Check sheet for the modelled part. Datum: model origin and axes. Units: mm. A direction names the side the tool comes from. Round coordinates to 2 decimals unless told otherwise and drop trailing zeros. Loops run counter-clockwise (first coordinate to the right, second up) from the corner with the lowest first, then second, coordinate; pieces in that order, holes last. Notation, with made-up numbers: (-8, 28) - (-3, 28) arc R20 cw to (-3, 39) - close; hole circle Ø10 at (-23.5, 68.25). An arc over 180 degrees is marked (long way). Return JSON: item names as keys, results as strings.
from build123d import *

# Parameters (mm, degrees)
PAD_DEPTH           = 26
SKETCH001_R         = 1.6891
POCKET_DEPTH        = 24.5
POCKET001_DEPTH     = 1.6
POCKET002_DEPTH     = 5
POCKET004_DEPTH     = 10
LINEARPATTERN_COUNT = 8
LINEARPATTERN_PITCH = 3.714286
SKETCH009_W         = 20
SKETCH009_H         = 4.8
POCKET007_DEPTH     = 0.5
SKETCH004_W         = 17.68
SKETCH004_H         = 4.4
POCKET015_DEPTH     = 5
SKETCH013_W         = 10.6
SKETCH013_H         = 6
POCKET016_DEPTH     = 5
SKETCH014_R         = 0.5
POCKET017_DEPTH     = 5
SKETCH015_R         = 1.9685
POCKET018_DEPTH     = 5
POCKET019_DEPTH     = 5
POCKET020_DEPTH     = 10
SKETCH021_R         = 7
PAD001_DEPTH        = 9
SKETCH019_R         = 4.6
POCKET021_DEPTH     = 1.2
SKETCH018_R         = 4
POCKET022_DEPTH     = 8.5


with BuildPart() as part:
    # Sketch → Pad (new body)
    with BuildSketch(Plane.XY):
        with BuildLine():
            Line((-17, 37.5), (17, 37.5))
            ThreePointArc((21, 33.5), (19.828427, 36.328427), (17, 37.5))
            Line((21, 33.5), (21, -33.5))
            ThreePointArc((17, -37.5), (19.828427, -36.328427), (21, -33.5))
            Line((17, -37.5), (-17, -37.5))
            ThreePointArc((-21, -33.5), (-19.828427, -36.328427), (-17, -37.5))
            Line((-21, -33.5), (-21, 33.5))
            ThreePointArc((-17, 37.5), (-19.828427, 36.328427), (-21, 33.5))
        make_face()
    extrude(amount=PAD_DEPTH)

    # Sketch001 (on Face10 of Pad) → Pocket (cut)
    with BuildSketch(Plane.XY.offset(26)):
        with Locations((-16.5, -33)):
            Circle(SKETCH001_R)
        with Locations((16.5, -33)):
            Circle(SKETCH001_R)
        with Locations((16.5, 33)):
            Circle(SKETCH001_R)
        with Locations((-16.5, 33)):
            Circle(SKETCH001_R)
        with BuildLine():
            Line((-12.6, 36), (12.6, 36))
            Line((12.6, 36), (12.6, 33.1))
            ThreePointArc((12.6, 33.1), (13.771573, 30.271573), (16.6, 29.1))
            Line((16.6, 29.1), (19.5, 29.1))
            Line((19.5, 29.1), (19.5, -29.1))
            Line((19.5, -29.1), (16.6, -29.1))
            ThreePointArc((16.6, -29.1), (13.771573, -30.271573), (12.6, -33.1))
            Line((12.6, -33.1), (12.6, -36))
            Line((12.6, -36), (-12.6, -36))
            Line((-12.6, -36), (-12.6, -33.1))
            ThreePointArc((-12.6, -33.1), (-13.771573, -30.271573), (-16.6, -29.1))
            Line((-16.6, -29.1), (-19.5, -29.1))
            Line((-19.5, -29.1), (-19.5, 29.1))
            Line((-19.5, 29.1), (-16.6, 29.1))
            ThreePointArc((-16.6, 29.1), (-13.771573, 30.271573), (-12.6, 33.1))
            Line((-12.6, 33.1), (-12.6, 36))
        make_face()
    extrude(amount=-POCKET_DEPTH, mode=Mode.SUBTRACT)

    # Sketch002 (on Face5 of Pocket) → Pocket001 (cut)
    with BuildSketch(Plane.XY.offset(26)):
        with BuildLine():
            Line((-17, 36), (17, 36))
            ThreePointArc((19.5, 33.5), (18.767767, 35.267767), (17, 36))
            Line((19.5, 33.5), (19.5, -33.5))
            ThreePointArc((17, -36), (18.767767, -35.267767), (19.5, -33.5))
            Line((17, -36), (-17, -36))
            ThreePointArc((-19.5, -33.5), (-18.767767, -35.267767), (-17, -36))
            Line((-19.5, -33.5), (-19.5, 33.5))
            ThreePointArc((-17, 36), (-18.767767, 35.267767), (-19.5, 33.5))
        make_face()
    extrude(amount=-POCKET001_DEPTH, mode=Mode.SUBTRACT)

    # Sketch003 (on Face7 of Pocket001) → Pocket002 (cut)
    with BuildSketch(Plane(origin=(0, 37.5, 0), x_dir=(-1, 0, 0), z_dir=(0, 1, 0))):
        with BuildLine():
            Line((5.4685, 16.5), (5.4685, 26))
            Line((5.4685, 26), (11.6915, 26))
            Line((11.6915, 26), (11.6915, 16.5))
            ThreePointArc((5.4685, 16.5), (8.58, 13.3885), (11.6915, 16.5))
        make_face()
    extrude(amount=-POCKET002_DEPTH, mode=Mode.SUBTRACT)

    # Sketch005 → Pocket004 (cut)
    with BuildSketch(Plane.XY.offset(1.5)):
        with BuildLine():
            ThreePointArc((-14, -25), (-13, -26), (-12, -25))
            Line((-12, -25), (-12, 6))
            ThreePointArc((-12, 6), (-13, 7), (-14, 6))
            Line((-14, -25), (-14, 6))
        make_face()
    pocket004 = extrude(amount=-POCKET004_DEPTH, mode=Mode.SUBTRACT)

    # LinearPattern: Pocket004 ×8
    with Locations(*[(i * LINEARPATTERN_PITCH, 0, 0) for i in range(1, LINEARPATTERN_COUNT)]):
        add(pocket004, mode=Mode.SUBTRACT)

    # Sketch009 → Pocket007 (cut)
    with BuildSketch(Plane(origin=(0, 37.5, 0), x_dir=(-1, 0, 0), z_dir=(0, 1, 0))):
        with Locations((-5.6, 18.9)):
            Rectangle(SKETCH009_W, SKETCH009_H)
    extrude(amount=-POCKET007_DEPTH, mode=Mode.SUBTRACT)

    # Sketch004 → Pocket015 (cut)
    with BuildSketch(Plane.YZ.offset(21)):
        with Locations((10.57, 23.8)):
            Rectangle(SKETCH004_W, SKETCH004_H)
    extrude(amount=-POCKET015_DEPTH, mode=Mode.SUBTRACT)

    # Sketch013 (on Face7 of Pocket007) → Pocket016 (cut)
    with BuildSketch(Plane(origin=(0, 37.5, 0), x_dir=(-1, 0, 0), z_dir=(0, 1, 0))):
        with Locations((-5.6, 18.9)):
            Rectangle(SKETCH013_W, SKETCH013_H)
    extrude(amount=-POCKET016_DEPTH, mode=Mode.SUBTRACT)

    # Sketch014 (on Face87 of Pocket016) → Pocket017 (cut)
    with BuildSketch(Plane(origin=(0, 37, 0), x_dir=(-1, 0, 0), z_dir=(0, 1, 0))):
        with Locations((-13.25, 18.9)):
            Circle(SKETCH014_R)
        with Locations((2.05, 18.9)):
            Circle(SKETCH014_R)
    extrude(amount=-POCKET017_DEPTH, mode=Mode.SUBTRACT)

    # Sketch015 (on Face104 of Pocket017) → Pocket018 (cut)
    with BuildSketch(Plane.XY.offset(24.4)):
        with Locations((-16.5, 33)):
            Circle(SKETCH015_R)
        with Locations((-16.5, -33)):
            Circle(SKETCH015_R)
        with Locations((16.5, -33)):
            Circle(SKETCH015_R)
        with Locations((16.5, 33)):
            Circle(SKETCH015_R)
    extrude(amount=-POCKET018_DEPTH, mode=Mode.SUBTRACT)

    # Sketch016 (on Face1 of Pocket018) → Pocket019 (cut)
    with BuildSketch(Plane(origin=(-21, 0, 0), x_dir=(0, -1, 0), z_dir=(-1, 0, 0))):
        with BuildLine():
            Line((-24.5, 26), (1.5, 26))
            Line((1.5, 26), (1.5, 15))
            ThreePointArc((-0.5, 13), (0.914214, 13.585786), (1.5, 15))
            Line((-0.5, 13), (-22.5, 13))
            ThreePointArc((-24.5, 15), (-23.914214, 13.585786), (-22.5, 13))
            Line((-24.5, 15), (-24.5, 26))
        make_face()
    extrude(amount=-POCKET019_DEPTH, mode=Mode.SUBTRACT)

    # Sketch020 (on Face81 of Pocket019) → Pocket020 (cut)
    with BuildSketch(Plane.XY.offset(1.5)):
        with BuildLine():
            Line((-19.5, 29.1), (-16.6, 29.1))
            ThreePointArc((-16.6, 29.1), (-13.771573, 30.271573), (-12.6, 33.1))
            Line((-12.6, 33.1), (-12.6, 36))
            Line((-12.6, 36), (12.6, 36))
            Line((12.6, 36), (12.6, 33.1))
            ThreePointArc((12.6, 33.1), (13.771573, 30.271573), (16.6, 29.1))
            Line((16.6, 29.1), (19.5, 29.1))
            Line((19.5, 29.1), (19.5, -33.5))
            ThreePointArc((17, -36), (18.767767, -35.267767), (19.5, -33.5))
            Line((17, -36), (-17, -36))
            ThreePointArc((-19.5, -33.5), (-18.767767, -35.267767), (-17, -36))
            Line((-19.5, -33.5), (-19.5, 29.1))
        make_face()
    extrude(amount=POCKET020_DEPTH, mode=Mode.SUBTRACT)

    # Sketch021 (on Face81 of Pocket020) → Pad001 (join)
    with BuildSketch(Plane.XY.offset(1.5)):
        with Locations((0, 25)):
            Circle(SKETCH021_R)
    extrude(amount=PAD001_DEPTH)

    # Sketch019 (on Face2 of Pad001) → Pocket021 (cut)
    with BuildSketch(Plane(origin=(0, 0, 0), x_dir=(1, 0, 0), z_dir=(0, 0, -1))):
        with Locations((0, -25)):
            Circle(SKETCH019_R)
    extrude(amount=-POCKET021_DEPTH, mode=Mode.SUBTRACT)

    # Sketch018 (on Face2 of Pad001) → Pocket022 (cut)
    with BuildSketch(Plane(origin=(0, 0, 0), x_dir=(1, 0, 0), z_dir=(0, 0, -1))):
        with Locations((0, -25)):
            Circle(SKETCH018_R)
    extrude(amount=-POCKET022_DEPTH, mode=Mode.SUBTRACT)


solid = part.part
Q1. Depth check by flat-ended pin: P1, Ø1.5, axis at x = -12, y = 19, coming from the +Z side; P2, Ø2, axis at x = 15.5, y = -32.5, coming from the +Z side; P3, Ø1.4, axis at x = 18.5, z = 16.5, coming from the +Y side. Enter the tip coordinate at first touch or a pass-through.
Answer key:
{"P1": "stops at z = 1.5", "P2": "stops at z = 24.4", "P3": "stops at y = 37.42"}
Q2. Tool access check on faces 1 (the face through (1.9, 7, 0.8)), 2 (the face through (20, 1.73, 24)), 3 (the face through (-20, -1.5, 21)). Record the directions out of +Z, -Z, +X, -X, +Y, -Y that give a thin tool (end or side, any length) a straight path to the whole face; none if there is none.
Answer key:
{"face 1": "+Z, -Z", "face 2": "+Z, +X, -X", "face 3": "+Z, -X"}
Q3. Sectioned sample at B-B (y = -22). State how many separate pieces and enclosed holes the cut face has, plus the area to 4 significant figures.
Answer key:
{"separate pieces": "9", "enclosed holes": "0", "area": "112.5 mm²"}
Q4. Draft check along Z on faces 4 (the face through (0, 25, 8.5)), 5 (the face through (10.9, 36.6, 18.9)), 6 (the face through (-4.571, -10, 1)). Enter one of: released by +Z, released by -Z, zero draft, split by the parting line, or undercut.
Answer key:
{"face 4": "released by -Z", "face 5": "undercut", "face 6": "zero draft"}
Q5. Sectioned sample at A-A (y = 10.5). Enter the section's corners in (x, z).
Answer key:
{"outline": "(-21, 0) - (21, 0) - (21, 21.6) - (19.5, 21.6) - (19.5, 1.5) - (-19.5, 1.5) - (-19.5, 13) - (-21, 13) - close"}
Q6. Scan lines: probe 1 along Y at (x, z) = (16.5, 22.35); probe 2 along Y at (x, z) = (-16.5, 16.25); probe 3 along X at (y, z) = (-28, 9). Record each from-to range of solid material in increasing order. Write a range as [from, to].
Answer key:
{"probe 1": "y = [-37.5, -34.97], [-31.03, -29.1], [29.1, 31.03], [34.97, 37.5]", "probe 2": "y = [-37.5, -34.69], [-31.31, -29.1], [29.1, 31.31], [34.69, 37.5]", "probe 3": "x = [-21, -19.5], [19.5, 21]"}
